from build123d import *

# Parameters (mm, degrees)
PAD_DEPTH         = 40
SKETCH001_W       = 4
SKETCH001_H       = 4.4
POCKET_DEPTH      = 0.001
POCKET_DEPTH_BACK = -40.001
FILLET_R          = 1
SKETCH002_R       = 1.6
POCKET001_DEPTH   = 3.001


with BuildPart() as part:
    # Sketch → Pad (new body)
    with BuildSketch(Plane.XY):
        Polygon((-12.5, -3), (-12.5, -18), (0, -5.5), (12.5, -18), (12.5, -3), (26, -3), (26, 0), (18, 0), (18, -1), (-18, -1), (-18, 0), (-26, 0), (-26, -3), align=None)
    extrude(amount=PAD_DEPTH)

    # Sketch001 → Pocket (cut, two sides)
    with BuildSketch(Plane.XY) as pocket_sk:
        with Locations((-10.5, -9.2)):
            Rectangle(SKETCH001_W, SKETCH001_H)
        with Locations((10.5, -9.2)):
            Rectangle(SKETCH001_W, SKETCH001_H)
    extrude(amount=-POCKET_DEPTH, mode=Mode.SUBTRACT)
    extrude(pocket_sk.sketch, amount=-POCKET_DEPTH_BACK, mode=Mode.SUBTRACT)

    # Fillet
    fillet_edges = [part.edges().sort_by_distance(p)[0] for p in [
        (-12.5, -18, 20),
        (12.5, -18, 20),
    ]]
    fillet(fillet_edges, radius=FILLET_R)

    # Sketch002 (on Face12 of Fillet) → Pocket001 (cut, through all)
    with BuildSketch(Plane.XZ.offset(3)):
        with Locations((-22, 5)):
            Circle(SKETCH002_R)
        with Locations((-22, 35)):
            Circle(SKETCH002_R)
        with Locations((22, 35)):
            Circle(SKETCH002_R)
        with Locations((22, 5)):
            Circle(SKETCH002_R)
    extrude(amount=-POCKET001_DEPTH, mode=Mode.SUBTRACT)


solid = part.part
Could you check a few things on this model? Use its own coordinates, in mm. A direction names the side the tool comes from. Coordinates: 2 decimals unless noted, no trailing zeros. Order: outer loops, then holes, each group sorted by start corner. A loop starts at its lowest first (then second) coordinate and runs counter-clockwise, first axis right, second up. Notation, with made-up numbers: (9.25, 53) -> (26.25, 53) arc R14 cw to (26.25, 79) -> close; hole circle Ø3 at (7.5, 16.25). An arc over 180 degrees is marked (long way). One line per item, written item: value. Start each with the question number.
1) Which directions (+Z, -Z, +X, -X, +Y, -Y) give clear straight access to the entire face, cutting with the end or side of a thin tool? Please do faces 5 (the flat face through (0, -1, 20)), 6 (the flat face through (5.3, -10.8, 19.7)), 7 (the flat face through (-12.5, -13, 20)), 8 (the flat face through (19, -3, 20)).
2) We'd pull the mould along Y, two halves only. Please class faces 1 (the flat face through (-11, -11.4, 20)), 2 (the cylindrical face through (-21.26, -1.52, 33.58)), 3 (the flat face through (-8.5, -9, 20)), 4 (the cylindrical face through (-11.867, -16.516, 20.28)): +Y half, -Y half, draft (parallel to the pull), parting line (faces both ways), or undercut.
3) Imagine slicing it at B-B on x = 9.5. List the corners of the cut face in (y, z) for me.
4) If I drill on L1, parallel to Z at x = -22, y = -2.2; L2, parallel to Y at x = 14, z = 9; L3, parallel to X at y = -7.5, z = 21, over which ranges is the centre line in solid material (lowest first)? Write a range as [from, to].
5) Imagine slicing it at C-C on z = 35. Count the separate pieces of the cut face and the enclosed holes in it, plus the area to 3 significant figures.
6) Imagine slicing it at A-A on y = -12.75. List the corners of the cut face in (x, z) for me, plus the area to 3 significant figures.
7) I'm going to push flat-ended pins straight in: pin 1 (3 mm diameter, centred on y = -5, z = 14, fed in from -X); pin 2 (11 mm diameter, centred on x = 9, z = 30, fed in from +Y); pin 3 (12 mm diameter, centred on x = 16, z = 5, fed in from -Y); pin 4 (4 mm diameter, centred on x = 20.5, z = 21, fed in from -Y). Where does each tip first touch, or does it pass through?
8) Imagine slicing it at D-D on x = -22. List the corners of the cut face in (y, z) for me, plus the area to 3 significant figures.
Answer list:
1. face 5: +Z, -Z, +Y
1. face 6: +Z, -Z, -Y
1. face 7: +Z, -Z, -X, -Y
1. face 8: +Z, -Z, +X, -Y
2. face 1: undercut
2. face 2: draft
2. face 3: undercut
2. face 4: -Y half
3. outline: (-15, 0) -> (-11.4, 0) -> (-11.4, 40) -> (-15, 40) -> close; (-7, 0) -> (-1, 0) -> (-1, 40) -> (-7, 40) -> close
4. L1: z = [0, 3.4], [6.6, 33.4], [36.6, 40]
4. L2: y = [-3, -1]
4. L3: x = [-8.5, -2], [2, 8.5]
5. separate pieces: 3
5. enclosed holes: 0
5. area: 282 mm2
6. outline: (-12.5, 0) -> (-7.25, 0) -> (-7.25, 40) -> (-12.5, 40) -> close; (7.25, 0) -> (12.5, 0) -> (12.5, 40) -> (7.25, 40) -> close
6. area: 420 mm2
7. pin 1: stops at x = -12.5
7. pin 2: stops at y = -1
7. pin 3: stops at y = -16.59
7. pin 4: stops at y = -3
8. outline: (-3, 0) -> (0, 0) -> (0, 3.4) -> (-3, 3.4) -> close; (-3, 6.6) -> (0, 6.6) -> (0, 33.4) -> (-3, 33.4) -> close; (-3, 36.6) -> (0, 36.6) -> (0, 40) -> (-3, 40) -> close
8. area: 101 mm2
